Input: part model. Units: mm. Frame: model coordinates. A direction names the side the tool comes from. Give positions to 0.01 mm unless a question says otherwise; leave off trailing zeros. Loops run counter-clockwise (first coordinate to the right, second up) from the corner with the lowest first, then second, coordinate; pieces in that order, holes last. Notation, with made-up numbers: (79, -39) - (116, -39) arc R21 cw to (116, -15) - close; hole circle Ø10 at (47.25, 82.25). An arc over 180 degrees is marked (long way). Answer as a JSON object with one key per item and string values. Group by question number.
(1) Pin query (flat end, axial travel): P1, Ø2, axis at x = -10.5, y = 3.5, coming from the -Z side; P2, Ø2, axis at x = 0, y = 8.5, coming from the +Z side; P3, Ø1, axis at x = 5.5, z = 3, coming from the +Y side; P4, Ø1, axis at x = 10, z = 2.5, coming from the -Y side. Return the tip coordinate at first contact, or that it passes through.
(2) Section query B-B (y = -8). Return loops of the section in (x, z).
(3) Section query C-C (x = 12). Return loops of the section in (y, z).
(4) Section query A-A (x = 0). Return loops of the section in (y, z).
(5) Access query for faces 1 (the flat face through (-4, -2, 1.6)), 2 (the cylindrical face through (5.9, 0.09, 3.51)), 3 (the cylindrical face through (-3.365, 13.066, 2.218)). Directions: +Z, -Z, +X, -X, +Y, -Y. A direction counts if a zero-diameter tool reaches every point of the face in a straight line with its end or side. Return the directions, or none.
(6) Section query D-D (y = -1.75). Return loops of the section in (x, z).
(7) Material intervals for L1, parallel to Y at x = 0, z = 3.15; L2, parallel to X at y = 1, z = 4.1; L3, parallel to Y at x = -1.5, z = 3, sorted ascending.
(8) Mould query, pull axis Y, two halves, no side actions, for faces 4 (the flat face through (-4, 4, 2.5)), 5 (the cylindrical face through (-14.985, 0.66, 2.218)), 6 (the flat face through (3, -10, 0)). Classes: +Y half, -Y half, draft (parallel to the pull), parting line (faces both ways), or undercut.
```python
from build123d import *

# Parameters (mm, degrees)
SKETCH_1_R          = 15
SKETCH_1_R_2        = 2.3
SKETCH_1_R_3        = 1.1
SKETCH_1_R_4        = 1
EXTRUDE_1_DEPTH     = 4.5
SKETCH_2_R          = 2.1
CUT_EXTRUDE_1_DEPTH = 2
SKETCH_10_R         = 10
CUT_EXTRUDE_7_DEPTH = 1.6
SKETCH_9_R          = 4.2
CUT_EXTRUDE_5_DEPTH = 3.9
SKETCH_6_R          = 1
CUT_EXTRUDE_6_DEPTH = 2


with BuildPart() as part:
    # 스케치1 → 보스-돌출1 (new body)
    with BuildSketch(Plane.XY):
        Circle(SKETCH_1_R)
        Circle(SKETCH_1_R_2, mode=Mode.SUBTRACT)
        with Locations((0, 8)):
            Circle(SKETCH_1_R_3, mode=Mode.SUBTRACT)
        with Locations((8, 0)):
            Circle(SKETCH_1_R_3, mode=Mode.SUBTRACT)
        with Locations((0, -8)):
            Circle(SKETCH_1_R_3, mode=Mode.SUBTRACT)
        with Locations((-8, 0)):
            Circle(SKETCH_1_R_3, mode=Mode.SUBTRACT)
        with Locations((-3.235238064, 12.074072829)):
            Circle(SKETCH_1_R_4, mode=Mode.SUBTRACT)
        with Locations((12.074072829, -3.235238064)):
            Circle(SKETCH_1_R_4, mode=Mode.SUBTRACT)
        with Locations((3.235238064, -12.074072829)):
            Circle(SKETCH_1_R_4, mode=Mode.SUBTRACT)
        with Locations((-12.074072829, 3.235238064)):
            Circle(SKETCH_1_R_4, mode=Mode.SUBTRACT)
    extrude(amount=EXTRUDE_1_DEPTH)

    # 스케치2 → 컷-돌출1 (cut)
    with BuildSketch(Plane.XY.offset(4.5)):
        with Locations((0, 8)):
            Circle(SKETCH_2_R)
        with Locations((8, 0)):
            Circle(SKETCH_2_R)
        with Locations((0, -8)):
            Circle(SKETCH_2_R)
        with Locations((-8, 0)):
            Circle(SKETCH_2_R)
    extrude(amount=-CUT_EXTRUDE_1_DEPTH, mode=Mode.SUBTRACT)

    # 스케치10 → 컷-돌출7 (cut)
    with BuildSketch(Plane(origin=(0, 0, 0), x_dir=(-1, 0, 0), z_dir=(0, 0, -1))):
        Circle(SKETCH_10_R)
    extrude(amount=-CUT_EXTRUDE_7_DEPTH, mode=Mode.SUBTRACT)

    # 스케치9 → 컷-돌출5 (cut, through all)
    with BuildSketch(Plane(origin=(0, 0, 1.6), x_dir=(-1, 0, 0), z_dir=(0, 0, -1))):
        Circle(SKETCH_9_R)
    extrude(amount=-CUT_EXTRUDE_5_DEPTH, mode=Mode.SUBTRACT)

    # 스케치6 → 컷-돌출6 (cut)
    with BuildSketch(Plane.XY.offset(4.5)):
        with Locations((-3.959797975, 3.959797975)):
            Circle(SKETCH_6_R)
        with Locations((3.959797975, -3.959797975)):
            Circle(SKETCH_6_R)
    extrude(amount=-CUT_EXTRUDE_6_DEPTH, mode=Mode.SUBTRACT)


solid = part.part
```
Recorded:
{
 "1": {"P1": "stops at z = 0", "P2": "stops at z = 2.5", "P3": "stops at y = 14.14", "P4": "stops at y = -11.61"},
 "2": {"outline": "(-12.69, 0) - (-6, 0) - (-6, 1.6) - (-1.1, 1.6) - (-1.1, 2.5) - (-2.1, 2.5) - (-2.1, 4.5) - (-12.69, 4.5) - close; (1.1, 1.6) - (6, 1.6) - (6, 0) - (12.69, 0) - (12.69, 4.5) - (2.1, 4.5) - (2.1, 2.5) - (1.1, 2.5) - close"},
 "3": {"outline": "(-9, 0) - (-4.23, 0) - (-4.23, 4.5) - (-9, 4.5) - close; (-2.24, 0) - (9, 0) - (9, 4.5) - (-2.24, 4.5) - close"},
 "4": {"outline": "(-15, 0) - (-10, 0) - (-10, 1.6) - (-9.1, 1.6) - (-9.1, 2.5) - (-10.1, 2.5) - (-10.1, 4.5) - (-15, 4.5) - close; (-6.9, 1.6) - (-4.2, 1.6) - (-4.2, 4.5) - (-5.9, 4.5) - (-5.9, 2.5) - (-6.9, 2.5) - close; (4.2, 1.6) - (6.9, 1.6) - (6.9, 2.5) - (5.9, 2.5) - (5.9, 4.5) - (4.2, 4.5) - close; (9.1, 1.6) - (10, 1.6) - (10, 0) - (15, 0) - (15, 4.5) - (10.1, 4.5) - (10.1, 2.5) - (9.1, 2.5) - close"},
 "5": {"face 1": "-Z", "face 2": "+Z", "face 3": "+Z, -Z"},
 "6": {"outline": "(-14.9, 0) - (-9.85, 0) - (-9.85, 1.6) - (-3.82, 1.6) - (-3.82, 4.5) - (-6.84, 4.5) - (-6.84, 2.5) - (-9.16, 2.5) - (-9.16, 4.5) - (-14.9, 4.5) - close; (3.82, 1.6) - (9.85, 1.6) - (9.85, 0) - (14.9, 0) - (14.9, 4.5) - (9.16, 4.5) - (9.16, 2.5) - (6.84, 2.5) - (6.84, 4.5) - (3.82, 4.5) - close"},
 "7": {"L1": "y = -15 to -10.1, -5.9 to -4.2, 4.2 to 5.9, 10.1 to 15", "L2": "x = -14.97 to -9.85, -6.15 to -4.08, 4.08 to 6.15, 9.85 to 14.97", "L3": "y = -14.92 to -9.47, -6.53 to -3.92, 3.92 to 6.53, 9.47 to 14.92"},
 "8": {"face 4": "undercut", "face 5": "parting line", "face 6": "draft"}
}
